CAD build for the part. Positions are in the model's coordinates, mm. A direction names the side the tool comes from. Round coordinates to 2 decimals unless told otherwise and drop trailing zeros. Loops run counter-clockwise (first coordinate to the right, second up) from the corner with the lowest first, then second, coordinate; pieces in that order, holes last. Notation, with made-up numbers: M 67,56.25 L 75,56.25 A11 cw 75,63.25 Z; hole C -17,88 d6. An arc over 180 degrees is marked long. Use one line per item in the form item = value.
from build123d import *

# Parameters (mm, degrees)
F0_W     = 310
F0_H     = 300
F1_DEPTH = 16
F2_W     = 5
F2_H     = 300
F3_DEPTH = 16.001
F4_W     = 50
F4_H     = 275
F5_DEPTH = 6.5
F7_D     = 6.8
F7_DEPTH = 20
F7_TIP   = 2.0429261047


with BuildPart() as f1:
    # F0 (on Front) → F1 (new body)
    with BuildSketch(Plane.XZ):
        Rectangle(F0_W, F0_H)
    extrude(amount=F1_DEPTH)

    # F2 (on face) → F3 (cut, through all)
    with BuildSketch(Plane.XZ.offset(16)):
        with Locations((152.5, 0)):
            Rectangle(F2_W, F2_H)
        with Locations((-152.5, 0)):
            Rectangle(F2_W, F2_H)
    extrude(amount=-F3_DEPTH, mode=Mode.SUBTRACT)

    # F4 (on face) → F5 (cut)
    with BuildSketch(Plane.XZ.offset(16)):
        with Locations((0, 12.5)):
            Rectangle(F4_W, F4_H)
    extrude(amount=-F5_DEPTH, mode=Mode.SUBTRACT)

    # F7
    with Locations(Plane.XZ.offset(16)):
        with Locations((-75, 100), (75, 100), (75, -100), (-75, -100)):
            Hole(F7_D / 2, depth=F7_DEPTH)
            with Locations((0, 0, -(F7_DEPTH + F7_TIP / 2))):  # 118° drill point
                Cone(0, F7_D / 2, F7_TIP, mode=Mode.SUBTRACT)


solid = f1.part
1. Pull direction X, two halves, no side cores. Call faces 3 (the face through (150, -8, -2)), 4 (the face through (-2, -8, 150)), 5 (the face through (-25, -13, 11)): +X half, -X half, draft (parallel to the pull), parting line (faces both ways), or undercut.
Completed:
face_3 = +X half
face_4 = draft
face_5 = undercut
2. Cut at B-B on x = -75. Write the cut outline in (y, z), and give its area (3 significant figures).
Completed:
outline = M -16,-150 L 0,-150 L 0,-103.4 L -16,-103.4 Z; M -16,-96.6 L 0,-96.6 L 0,96.6 L -16,96.6 Z; M -16,103.4 L 0,103.4 L 0,150 L -16,150 Z
area = 4,580 mm2
3. Tool access for faces 1 (the face through (77.698, -7.888, -102.069)), 2 (the face through (0, -13, -125)): list every direction of +Z, -Z, +X, -X, +Y, -Y with a clear straight run to the whole face (end or side of a thin tool).
Completed:
face_1 = +Y, -Y
face_2 = +Z, -Y
4. Probe line 1 along Z through (x, y) = (75, -4.25); line 2 along Z through (x, y) = (-78, -8.5); line 3 along Y through (x, z) = (4.5, 97.5). List the from-to ranges inside material, lowest first. Write a range as from..to.
Completed:
line_1 = -150..-103.4, -96.6..96.6, 103.4..150
line_2 = -150..-101.6, -98.4..98.4, 101.6..150
line_3 = -9.5..0
5. Cut at A-A on z = 100. Write the cut outline in (x, y).
Completed:
outline = M -150,-16 L -78.4,-16 L -78.4,0 L -150,0 Z; M -71.6,-16 L -25,-16 L -25,-9.5 L 25,-9.5 L 25,-16 L 71.6,-16 L 71.6,0 L -71.6,0 Z; M 78.4,-16 L 150,-16 L 150,0 L 78.4,0 Z
